Geometry check sheet. Reference: the model listing, model coordinates, mm. Face numbers are marked on the shaded views. A direction names the side the tool comes from. Round coordinates to 2 decimals unless told otherwise and drop trailing zeros. Order: outer loops, then holes, each group sorted by start corner. A loop starts at its lowest first (then second) coordinate and runs counter-clockwise, first axis right, second up. Notation, with made-up numbers: (57, -13.75) - (70, -13.75) arc R22 cw to (70, 25.25) - close; hole circle Ø7 at (-10.75, 70). An arc over 180 degrees is marked (long way). Use a Markdown table: item, result. Add a question column.
(1) Thickness scan on line 1 along Y through (x, z) = (3.5, 0.75); line 2 along Z through (x, y) = (0.5, 1.25); line 3 along X through (y, z) = (4.8, 0). Record the ranges inside material, lowest first. Write a range as [from, to].
(2) Section check B-B on x = -2.25. Record the boundary of the cut face in (y, z).
(3) Section check C-C on y = -2.75. Record the boundary of the cut face in (x, z).
(4) Section check A-A on z = -2.25. Record the boundary of the cut face in (x, y), then the cut area to 3 significant figures.
(5) Section check D-D on z = 0. Record the boundary of the cut face in (x, y).
(6) Mould release check, pull along Y, two halves, no side actions. Record for the marked faces 1, 2 and 3: released by +Y, released by -Y, zero draft, split by the parting line, or undercut.
(7) Access from +Z, -Z, +X, -X, +Y, -Y to the whole of each face (thin tool, end or side, straight path). Record for the marked faces 4, 5 and 6.
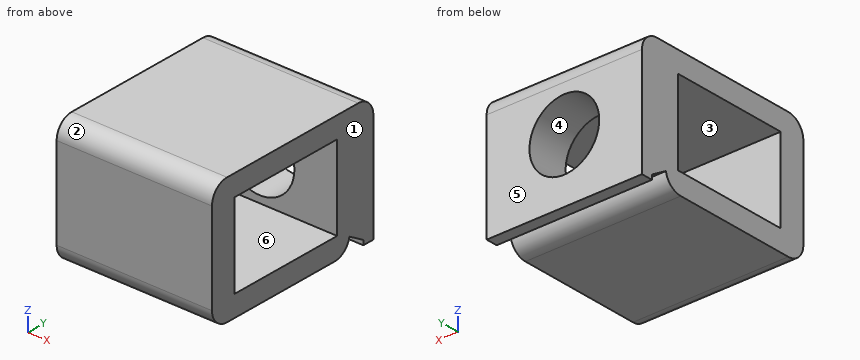
```python
from build123d import *

# Parameters (mm, degrees)
EXTRUDE_1_DEPTH      = 4.45
EXTRUDE_1_DEPTH_BACK = 4.45
SKETCH_1_W           = 7.2
SKETCH_1_H           = 10.7
SKETCH_1_W_2         = 4.8
SKETCH_1_H_2         = 6.8
SKETCH_2_R           = 2
CUT_EXTRUDE_1_DEPTH  = 5
CUT_EXTRUDE_2_DEPTH  = 8.9
FILLET_1_R           = 1


with BuildPart() as part:
    # 草图1 → 凸台-拉伸1 (new, two sides: drawn at the far end of the back side and taken through both)
    with BuildSketch(Plane(origin=(0, 0, 0), x_dir=(0, 0, -1), z_dir=(1, 0, 0)).offset(-EXTRUDE_1_DEPTH_BACK)):
        Rectangle(SKETCH_1_W, SKETCH_1_H)
        with Locations((0, -0.45)):
            Rectangle(SKETCH_1_W_2, SKETCH_1_H_2, mode=Mode.SUBTRACT)
    extrude(amount=EXTRUDE_1_DEPTH + EXTRUDE_1_DEPTH_BACK)

    # 草图2 → 切除-拉伸1 (cut)
    with BuildSketch(Plane(origin=(0, 5.35, 0), x_dir=(1, 0, 0), z_dir=(0, 1, 0))):
        with Locations(Location((0, 0, 0), (0, 0, 270))):
            Circle(SKETCH_2_R)
    extrude(amount=-CUT_EXTRUDE_1_DEPTH, mode=Mode.SUBTRACT)

    # 草图3 → 切除-拉伸2 (cut)
    with BuildSketch(Plane(origin=(4.45, 0, 0), x_dir=(0, 0, -1), z_dir=(1, 0, 0))):
        Polygon((3.6, 4.688566818), (3.336866457, 4.688566818), (2.775968401, 3.765242325), (3.6, 3.765242325), align=None)
    extrude(amount=-CUT_EXTRUDE_2_DEPTH, mode=Mode.SUBTRACT)

    # 圆角1
    # the kernel refuses this fillet: 1 mm, written as the material it takes off along each edge
    with BuildSketch(Plane(origin=(6.95, -5.35, -3.6), x_dir=(0, 0, 1), z_dir=(-1, 0, 0))) as fillet_1_piece_1:
        with BuildLine():
            CenterArc((FILLET_1_R, FILLET_1_R), FILLET_1_R, 180, 90)
            Line((0, FILLET_1_R), (-FILLET_1_R * 0.02, FILLET_1_R))
            Line((-FILLET_1_R * 0.02, FILLET_1_R), (-FILLET_1_R * 0.02, -FILLET_1_R * 0.02))
            Line((-FILLET_1_R * 0.02, -FILLET_1_R * 0.02), (FILLET_1_R, -FILLET_1_R * 0.02))
            Line((FILLET_1_R, -FILLET_1_R * 0.02), (FILLET_1_R, 0))
        make_face()
    extrude(amount=13.9, mode=Mode.SUBTRACT)
    with BuildSketch(Plane(origin=(-6.95, -5.35, 3.6), x_dir=(0, 1, 0), z_dir=(1, 0, 0)), Plane(origin=(-6.95, 5.35, 3.6), x_dir=(0, 0, -1), z_dir=(1, 0, 0))) as fillet_1_piece_2:
        with BuildLine():
            CenterArc((FILLET_1_R, -FILLET_1_R), FILLET_1_R, 90, 90)
            Line((0, -FILLET_1_R), (-FILLET_1_R * 0.02, -FILLET_1_R))
            Line((-FILLET_1_R * 0.02, -FILLET_1_R), (-FILLET_1_R * 0.02, FILLET_1_R * 0.02))
            Line((-FILLET_1_R * 0.02, FILLET_1_R * 0.02), (FILLET_1_R, FILLET_1_R * 0.02))
            Line((FILLET_1_R, FILLET_1_R * 0.02), (FILLET_1_R, 0))
        make_face()
    extrude(amount=13.9, mode=Mode.SUBTRACT)
    with BuildSketch(Plane(origin=(6.910989539, 3.765242325, -3.6), x_dir=(0, -1, 0), z_dir=(-1, 0, 0))) as fillet_1_piece_3_section:
        with BuildLine():
            CenterArc((0.984395816, 1), FILLET_1_R, 190.135017985, 79.864982015)
            Line((0, 0.824031599), (-0.019687916, 0.820512231))
            ThreePointArc((-0.019687916, 0.820512231), (-0.02, 0.412015799), (-0.02, 0))
            Line((-0.02, 0), (0, -0.02))
            Line((0, -0.02), (0.984395816, -0.02))
            Line((0.984395816, -0.02), (0.984395816, 0))
        make_face()
    fillet_1_piece_3 = extrude(amount=13.821979078, mode=Mode.PRIVATE)
    fillet_1_piece_3 = split(fillet_1_piece_3, bisect_by=Plane(origin=(0, 3.873370959, -2.84165402), z_dir=(0, -0.5191865527287748, -0.8546609406458278)), keep=Keep.TOP, mode=Mode.PRIVATE)
    add(fillet_1_piece_3, mode=Mode.SUBTRACT)


solid = part.part
```
Check sheet entries:
| question | item | result |
|---|---|---|
| 1 | line 1 | y = [-5.35, -3.85], [2.95, 5.35] |
| 1 | line 2 | z = [-3.6, -2.4], [2.4, 3.6] |
| 1 | line 3 | x = [-4.45, -2], [2, 4.45] |
| 2 | outline | (-5.35, -2.6) arc R1 ccw to (-4.35, -3.6) - (2.78, -3.6) arc R1 ccw to (3.77, -2.78) - (4.69, -3.34) - (4.69, -3.6) - (5.35, -3.6) - (5.35, 2.6) arc R1 ccw to (4.35, 3.6) - (-4.35, 3.6) arc R1 ccw to (-5.35, 2.6) - close; hole (-3.85, -2.4) - (2.95, -2.4) - (2.95, 2.4) - (-3.85, 2.4) - close |
| 3 | outline | (-4.45, -3.6) - (4.45, -3.6) - (4.45, -2.4) - (-4.45, -2.4) - close; (-4.45, 2.4) - (4.45, 2.4) - (4.45, 3.6) - (-4.45, 3.6) - close |
| 4 | outline | (-4.45, -5.35) - (4.45, -5.35) - (4.45, -3.85) - (-4.45, -3.85) - close; (-4.45, 2.95) - (4.45, 2.95) - (4.45, 5.35) - (-4.45, 5.35) - close |
| 4 | area | 34.7 mm2 |
| 5 | outline | (-4.45, -5.35) - (4.45, -5.35) - (4.45, -3.85) - (-4.45, -3.85) - close; (-4.45, 2.95) - (-2, 2.95) - (-2, 5.35) - (-4.45, 5.35) - close; (2, 2.95) - (4.45, 2.95) - (4.45, 5.35) - (2, 5.35) - close |
| 6 | face 1 | zero draft |
| 6 | face 2 | released by -Y |
| 6 | face 3 | undercut |
| 7 | face 4 | +Y |
| 7 | face 5 | +Z, -Z, +X, -X, +Y |
| 7 | face 6 | +X, -X |
